The model under review builds one solid part; all positions refer to its coordinate system, in mm. Face numbers are marked on the shaded views. A direction names the side the tool comes from. Round coordinates to 2 decimals unless told otherwise and drop trailing zeros. Order: outer loops, then holes, each group sorted by start corner. A loop starts at its lowest first (then second) coordinate and runs counter-clockwise, first axis right, second up. Notation, with made-up numbers: (49.5, 85.5) -> (56.5, 85.5) arc R32 ccw to (56.5, 114.5) -> close; hole circle Ø7 at (26, 32.25). An arc over 180 degrees is marked (long way). Use a Markdown table: item, result. Add a question column.
```python
from build123d import *

# Parameters (mm, degrees)
F0_R     = 10
F1_DEPTH = 6.35
F3_DEPTH = 25.4
F5_DEPTH = 25.4
F6_R     = 2.859513
F7_DEPTH = 25.4


with BuildPart() as f1:
    # F0 (on Front) → F1 (new body)
    with BuildSketch(Plane.XZ):
        Circle(F0_R)
    extrude(amount=F1_DEPTH)

    # F2 (on Front) → F3 (cut)
    with BuildSketch(Plane.XZ):
        with BuildLine():
            Line((5.17427, 1.104157), (-6.035211, 1.104157))
            ThreePointArc((-6.035211, 1.104157), (-7.016857, 0.122512), (-6.035211, -0.859134))
            Line((-6.035211, -0.859134), (5.17427, -0.859134))
            ThreePointArc((5.17427, -0.859134), (6.155916, 0.122512), (5.17427, 1.104157))
        make_face()
    extrude(amount=F3_DEPTH, mode=Mode.SUBTRACT)

    # F4 (on Front) → F5 (cut)
    with BuildSketch(Plane.XZ):
        with BuildLine():
            Line((1.099834, -2.258694), (1.099834, 0))
            Line((1.099834, 0), (1.099834, 2.258694))
            ThreePointArc((1.099834, 2.258694), (-0.000652, 2.419633), (-1.101137, 2.258694))
            Line((-1.101137, 2.258694), (-1.101137, 0))
            Line((-1.101137, 0), (-1.101137, -2.258694))
            ThreePointArc((-1.101137, -2.258694), (-0.000652, -2.419633), (1.099834, -2.258694))
        make_face()
    extrude(amount=F5_DEPTH, mode=Mode.SUBTRACT)

    # F6 (on face) → F7 (cut)
    with BuildSketch(Plane.XZ.offset(6.35)):
        with Locations((-3.97266, 4.139036)):
            Circle(F6_R)
        with Locations((-3.97266, -4.139036)):
            Circle(F6_R)
        with Locations((3.972278, 4.138778)):
            Circle(F6_R)
        with Locations((3.971739, -4.139295)):
            Circle(F6_R)
    extrude(amount=-F7_DEPTH, mode=Mode.SUBTRACT)


solid = f1.part
```
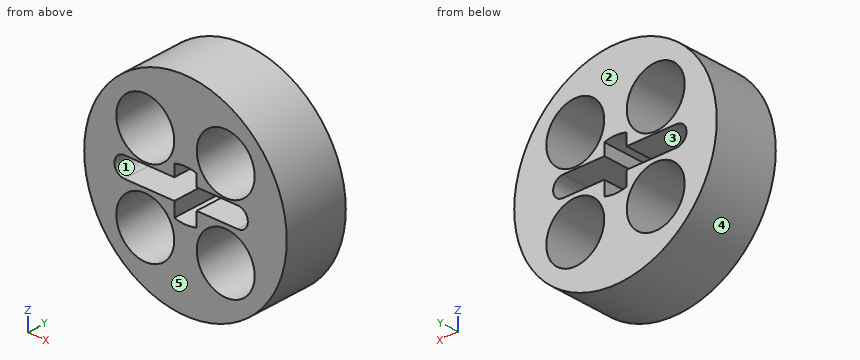
Q1. Add section A-A (x = 0). Write out the cut boundary in (y, z), then the cut area to 3 significant figures.
Q2. Wall thickness on line 1 (Z direction, x = 4, y = -5.25); line 2 (X direction, y = -4.5, z = -4.75); line 3 (X direction, y = -1.75, z = -4): over which ranges is each line inside the solid? List them lowest first. Write a range as [from, to].
Q3. Add section C-C (z = 0). Write out the cut boundary in (x, y).
Q4. Insertion check: pin 1 (1.3 mm diameter, centred on y = -3, z = 2, fed in from -X); pin 2 (1.1 mm diameter, centred on y = -2.5, z = -1, fed in from -X); pin 3 (3.5 mm diameter, centred on x = 3.5, y = -2, fed in from -Z). Each pin has a flat end and moves straight along its axis. Give the tip position at first contact, or say it passes through.
Q5. Add section B-B (x = 5.5). Write out the cut boundary in (y, z), then the cut area to 3 significant figures.
Q6. Mouldability with a two-part tool opening along Z and no side actions: class the marked faces 3, 4 and 5 as pulls with the +Z half, pulls with the -Z half, needs draft (parallel to the pull), parting line crosses it, or undercut.
Q7. Machinability: for the marked faces 1 and 2, which of the approach directions +Z, -Z, +X, -X, +Y, -Y give a long, thin tool a straight path to every point of the face, cutting with its end or side? Answer none if there is none.
Q8. Add section D-D (z = 5.25). Write out the cut boundary in (x, y).
Report:
| question | item | result |
|---|---|---|
| 1 | outline | (-6.35, -10) -> (0, -10) -> (0, -2.42) -> (-6.35, -2.42) -> close; (-6.35, 2.42) -> (0, 2.42) -> (0, 10) -> (-6.35, 10) -> close |
| 1 | area | 96.3 mm² |
| 2 | line 1 | z = [-9.17, -7], [-1.28, -0.86], [1.1, 1.28], [7, 9.17] |
| 2 | line 2 | x = [-8.8, -6.77], [-1.18, 1.18], [6.77, 8.8] |
| 2 | line 3 | x = [-9.17, -6.83], [-1.12, 1.12], [6.83, 9.17] |
| 3 | outline | (-10, -6.35) -> (-7.01, -6.35) -> (-7.01, 0) -> (-10, 0) -> close; (6.15, -6.35) -> (10, -6.35) -> (10, 0) -> (6.15, 0) -> close |
| 4 | pin 1 | stops at x = -9.91 |
| 4 | pin 2 | stops at x = -9.99 |
| 4 | pin 3 | stops at z = -9.85 |
| 5 | outline | (-6.35, -8.35) -> (0, -8.35) -> (0, -6.56) -> (-6.35, -6.56) -> close; (-6.35, -1.72) -> (0, -1.72) -> (0, -0.8) -> (-6.35, -0.8) -> close; (-6.35, 1.05) -> (0, 1.05) -> (0, 1.72) -> (-6.35, 1.72) -> close; (-6.35, 6.56) -> (0, 6.56) -> (0, 8.35) -> (-6.35, 8.35) -> close |
| 5 | area | 32.9 mm² |
| 6 | face 3 | undercut |
| 6 | face 4 | parting line crosses it |
| 6 | face 5 | needs draft |
| 7 | face 1 | +Y, -Y |
| 7 | face 2 | +Z, -Z, +X, -X, +Y |
| 8 | outline | (-8.51, -6.35) -> (-6.61, -6.35) -> (-6.61, 0) -> (-8.51, 0) -> close; (-1.34, -6.35) -> (1.34, -6.35) -> (1.34, 0) -> (-1.34, 0) -> close; (6.61, -6.35) -> (8.51, -6.35) -> (8.51, 0) -> (6.61, 0) -> close |
